The listing builds one solid part. Answer for the finished solid, in the listing's coordinates (mm). A direction names the side the tool comes from. Give positions to 0.01 mm unless a question says otherwise; leave off trailing zeros. Order: outer loops, then holes, each group sorted by start corner. A loop starts at its lowest first (then second) coordinate and runs counter-clockwise, first axis right, second up. Notation, with made-up numbers: (69, 34.25) - (110, 34.25) arc R7 cw to (110, 45.25) - close; hole circle Ø7 at (-14, 84). An arc over 180 degrees is marked (long way). Answer as a JSON object with one key per item and string values. Group by question number.
Q1. A cutting plane is placed at B-B, the plane x = 11. Give the vertices of the cut face in (y, z).
Q2. The mould has two halves that part along X. Classify faces 1 (the face through (12, 21, -15)), 2 (the face through (0, 21, -7)), 3 (the face through (9.755, 44.479, -6.791)), 4 (the face through (17, 43, -8)): released by +X, released by -X, zero draft, split by the parting line, or undercut.
Q3. Consider line 1 (X direction, y = 45.8, z = -7.5); line 2 (Y direction, x = 19, z = -9); line 3 (X direction, y = 45.5, z = -6). Determine where each line is inside the solid, lowest interval first.
Q4. For faces 5 (the face through (19.897, 44.38, -8.779)), 6 (the face through (12, 21, 0)), determine the directions among +Z, -Z, +X, -X, +Y, -Y from which every point of the face is accessible in a straight line to the end or side of a thin tool.
Q5. A cutting plane is placed at C-C, the plane z = -2.75. Give the vertices of the cut face in (x, y).
Q6. Given pin 1 (2.5 mm diameter, centred on x = 17.5, z = -7.5, fed in from +Y); pin 2 (1.5 mm diameter, centred on x = 19.5, z = -10, fed in from +Y), each flat-ended and moving along its own axis, determine where each tip first touches the part or whether it passes through.
from build123d import *

# Parameters (mm, degrees)
CROQUIS1_W              = 24
CROQUIS1_H              = 15
SALIENTE_EXTRUIR1_DEPTH = 43
CROQUIS2_R              = 2.771687151
CROQUIS2_R_2            = 2.271687151
CROQUIS2_R_3            = 3.271687151
SALIENTE_EXTRUIR2_DEPTH = 3
CROQUIS3_R              = 3.771687151
CROQUIS3_R_2            = 2.771687151
SALIENTE_EXTRUIR3_DEPTH = 1
REDONDEO1_R             = 0.4
REDONDEO2_R             = 0.2


with BuildPart() as part:
    # Croquis1 → Saliente-Extruir1 (new body)
    with BuildSketch(Plane(origin=(0, 0, 0), x_dir=(1, 0, 0), z_dir=(0, 1, 0))):
        with Locations((12, 7.5)):
            Rectangle(CROQUIS1_W, CROQUIS1_H)
    extrude(amount=SALIENTE_EXTRUIR1_DEPTH)

    # Croquis2 → Saliente-Extruir2 (add)
    # profile 1 of 2: a face of its own
    with BuildSketch(Plane(origin=(0, 43, 0), x_dir=(1, 0, 0), z_dir=(0, 1, 0))):
        with Locations(Location((17.438401582, 7.5, 0), (0, 0, 90))):
            Circle(CROQUIS2_R)
        with Locations(Location((17.438401582, 7.5, 0), (0, 0, 90))):
            Circle(CROQUIS2_R_2, mode=Mode.SUBTRACT)
    # profile 2 of 2: a face of its own
    with BuildSketch(Plane(origin=(0, 43, 0), x_dir=(1, 0, 0), z_dir=(0, 1, 0))):
        with Locations(Location((6.561598418, 7.5, 0), (0, 0, 90))):
            Circle(CROQUIS2_R_3)
        with Locations(Location((6.561598418, 7.5, 0), (0, 0, 270))):
            Circle(CROQUIS2_R, mode=Mode.SUBTRACT)
    extrude(amount=SALIENTE_EXTRUIR2_DEPTH)

    # Croquis3 → Saliente-Extruir3 (add)
    with BuildSketch(Plane(origin=(0, 46, 0), x_dir=(1, 0, 0), z_dir=(0, 1, 0))):
        with Locations(Location((6.561598418, 7.5, 0), (0, 0, 270))):
            Circle(CROQUIS3_R)
        with Locations(Location((6.561598418, 7.5, 0), (0, 0, 270))):
            Circle(CROQUIS3_R_2, mode=Mode.SUBTRACT)
    extrude(amount=SALIENTE_EXTRUIR3_DEPTH)

    # Redondeo1
    redondeo1_edges = [part.edges().sort_by_distance(p)[0] for p in [
        (6.561598418, 47, -11.271687151),
        (6.561598418, 46, -11.271687151),
        (6.561598418, 47, -10.271687151),
    ]]
    fillet(redondeo1_edges, radius=REDONDEO1_R)

    # Redondeo2
    redondeo2_edges = [part.edges().sort_by_distance(p)[0] for p in [
        (17.438401582, 46, -4.728312849),
        (17.438401582, 46, -5.228312849),
    ]]
    fillet(redondeo2_edges, radius=REDONDEO2_R)


solid = part.part
Reply:
{
 "1": {"outline": "(0, -15) - (43, -15) - (43, 0) - (0, 0) - close"},
 "2": {"face 1": "zero draft", "face 2": "released by -X", "face 3": "undercut", "face 4": "undercut"},
 "3": {"line 1": "x = 3.29 to 3.79, 9.33 to 9.83, 14.67 to 15.17, 19.71 to 20.21", "line 2": "y = 0 to 43", "line 3": "x = 3.65 to 4.23, 8.89 to 9.47, 15.11 to 15.73, 19.14 to 19.77"},
 "4": {"face 5": "+Y", "face 6": "+Z, +X, -X, +Y, -Y"},
 "5": {"outline": "(0, 0) - (24, 0) - (24, 43) - (0, 43) - close"},
 "6": {"pin 1": "stops at y = 43", "pin 2": "stops at y = 46"}
}
